```python
from build123d import *

# Parameters (mm, degrees)
BOSS_EXTRUDE1_DEPTH = 3


with BuildPart() as part:
    # Sketch1 → Boss-Extrude1 (new, symmetric)
    with BuildSketch(Plane(origin=(0, 0, 0), x_dir=(0, 0, -1), z_dir=(1, 0, 0))):
        with BuildLine():
            ThreePointArc((185, 90.5), (184.414213562, 91.914213562), (183, 92.5))
            Line((183, 92.5), (155, 92.5))
            ThreePointArc((155, 92.5), (133.786796564, 83.713203436), (125, 62.5))
            Line((125, 62.5), (125, 47.5))
            ThreePointArc((125, 47.5), (101.568542495, -9.068542495), (45, -32.5))
            Line((45, -32.5), (-155, -32.5))
            ThreePointArc((-155, -32.5), (-176.213203436, -41.286796564), (-185, -62.5))
            Line((-185, -62.5), (-185, -92.5))
            Line((-185, -92.5), (-176, -92.5))
            Line((-176, -92.5), (-176, -98.5))
            Line((-176, -98.5), (-166, -98.5))
            Line((-166, -98.5), (-166, -92.5))
            Line((-166, -92.5), (-149, -92.5))
            Line((-149, -92.5), (-149, -77.5))
            Line((-149, -77.5), (-150.7, -77.5))
            Line((-150.7, -77.5), (-150.7, -72))
            Line((-150.7, -72), (-149, -72))
            Line((-149, -72), (-149, -62))
            Line((-149, -62), (-142, -62))
            Line((-142, -62), (-142, -72))
            Line((-142, -72), (-140.3, -72))
            Line((-140.3, -72), (-140.3, -77.5))
            Line((-140.3, -77.5), (-142, -77.5))
            Line((-142, -77.5), (-142, -92.5))
            Line((-142, -92.5), (-125, -92.5))
            Line((-125, -92.5), (-125, -98.5))
            Line((-125, -98.5), (-115, -98.5))
            Line((-115, -98.5), (-115, -92.5))
            Line((-115, -92.5), (-30.5, -92.5))
            Line((-30.5, -92.5), (-30.5, -98.5))
            Line((-30.5, -98.5), (-20.5, -98.5))
            Line((-20.5, -98.5), (-20.5, -92.5))
            Line((-20.5, -92.5), (-3.5, -92.5))
            Line((-3.5, -92.5), (-3.5, -77.5))
            Line((-3.5, -77.5), (-5.2, -77.5))
            Line((-5.2, -77.5), (-5.2, -72))
            Line((-5.2, -72), (-3.5, -72))
            Line((-3.5, -72), (-3.5, -62))
            Line((-3.5, -62), (3.5, -62))
            Line((3.5, -62), (3.5, -72))
            Line((3.5, -72), (5.2, -72))
            Line((5.2, -72), (5.2, -77.5))
            Line((5.2, -77.5), (3.5, -77.5))
            Line((3.5, -77.5), (3.5, -92.5))
            Line((3.5, -92.5), (20.5, -92.5))
            Line((20.5, -92.5), (20.5, -98.5))
            Line((20.5, -98.5), (30.5, -98.5))
            Line((30.5, -98.5), (30.5, -92.5))
            Line((30.5, -92.5), (115, -92.5))
            Line((115, -92.5), (115, -98.5))
            Line((115, -98.5), (125, -98.5))
            Line((125, -98.5), (125, -92.5))
            Line((125, -92.5), (142, -92.5))
            Line((142, -92.5), (142, -77.5))
            Line((142, -77.5), (140.3, -77.5))
            Line((140.3, -77.5), (140.3, -72))
            Line((140.3, -72), (142, -72))
            Line((142, -72), (142, -62))
            Line((142, -62), (149, -62))
            Line((149, -62), (149, -72))
            Line((149, -72), (150.7, -72))
            Line((150.7, -72), (150.7, -77.5))
            Line((150.7, -77.5), (149, -77.5))
            Line((149, -77.5), (149, -92.5))
            Line((149, -92.5), (166, -92.5))
            Line((166, -92.5), (166, -98.5))
            Line((166, -98.5), (176, -98.5))
            Line((176, -98.5), (176, -92.5))
            Line((176, -92.5), (185, -92.5))
            Line((185, -92.5), (185, -73))
            ThreePointArc((185, -73), (184.414213562, -71.585786438), (183, -71))
            Line((183, -71), (182, -71))
            ThreePointArc((182, -71), (180.585786438, -70.414213562), (180, -69))
            Line((180, -69), (180, 67))
            ThreePointArc((180, 67), (180.585786438, 68.414213562), (182, 69))
            Line((182, 69), (183, 69))
            ThreePointArc((183, 69), (184.414213562, 69.585786438), (185, 71))
            Line((185, 71), (185, 90.5))
        make_face()
    extrude(amount=BOSS_EXTRUDE1_DEPTH, both=True)


solid = part.part
```
The model under review builds one solid part; all positions refer to its coordinate system, in mm. Round coordinates to 2 decimals unless told otherwise and drop trailing zeros. Loops run counter-clockwise (first coordinate to the right, second up) from the corner with the lowest first, then second, coordinate; pieces in that order, holes last. Notation, with made-up numbers: (41, 34.5) -> (89, 34.5) arc R22 ccw to (89, 63.5) -> close; hole circle Ø3 at (-40, 34.25). An arc over 180 degrees is marked (long way). Answer as a JSON object with one key per item and string values. Group by question number.
1) For pin 1 Ø1.8 at (x, z) = (0, -161) entering from -Y; pin 2 Ø1 at (x, z) = (2.5, 1.5) entering from +Y; pin 3 Ø1.5 at (x, y) = (1.5, -5) entering from +Z, all flat-tipped, find the tip position at first contact; note any pin that passes through.
2) We need section B-B on z = -109. Write out the cut boundary in (x, y), then the cut area to 3 significant figures.
3) We need section A-A on y = 53. Write out the cut boundary in (x, z), then the cut area to 3 significant figures.
4) For line 1 (Z direction, x = 1.45, y = -69); line 2 (Z direction, x = 1.5, y = -78); line 3 (Y direction, x = -1.6, z = 112.5), list the stretches that pass through material, from the lowest coordinate up. Write a range as [from, to].
5) Mouldability with a two-part tool opening along Y and no side actions: class faces 1 (the face through (0.04, -8.44, -102.19)), 2 (the face through (3, -44, -39)) as released by +Y, released by -Y, zero draft, split by the parting line, or undercut.
Result set:
{
 "1": {"pin 1": "y = -92.5", "pin 2": "y = -32.5", "pin 3": "z = -104.7"},
 "2": {"outline": "(-3, -92.5) -> (3, -92.5) -> (3, -0.5) -> (-3, -0.5) -> close", "area": "552 mm²"},
 "3": {"outline": "(-3, -180) -> (3, -180) -> (3, -125) -> (-3, -125) -> close", "area": "330 mm²"},
 "4": {"line 1": "[-180, -149], [-142, -3.5], [3.5, 142], [149, 185]", "line 2": "[-185, -149], [-142, -3.5], [3.5, 142], [149, 185]", "line 3": "[-92.5, -32.5]"},
 "5": {"face 1": "released by +Y", "face 2": "zero draft"}
}
